from build123d import *

# Parameters (mm, degrees)
SKETCH_R         = 1.65
EXTRUDE_DEPTH    = 5
SKETCH001_W      = 50.041317
SKETCH001_H      = 10.034617
EXTRUDE001_DEPTH = 5


with BuildPart() as extrude_body:
    # Sketch → Extrude (new body)
    with BuildSketch(Plane.XY):
        Circle(SKETCH_R)
        with Locations((-10, 0)):
            Circle(SKETCH_R)
        with Locations((-20, 0)):
            Circle(SKETCH_R)
        with Locations((10, 0)):
            Circle(SKETCH_R)
        with Locations((20, 0)):
            Circle(SKETCH_R)
    extrude(amount=EXTRUDE_DEPTH)


with BuildPart() as cut:
    # Sketch001 → Extrude001 (new body)
    with BuildSketch(Plane.XY):
        with Locations((-0.018242, 0.017349)):
            Rectangle(SKETCH001_W, SKETCH001_H)
    extrude(amount=EXTRUDE001_DEPTH)

    # Cut: cut Extrude body
    add(extrude_body.part, mode=Mode.SUBTRACT)


solid = cut.part
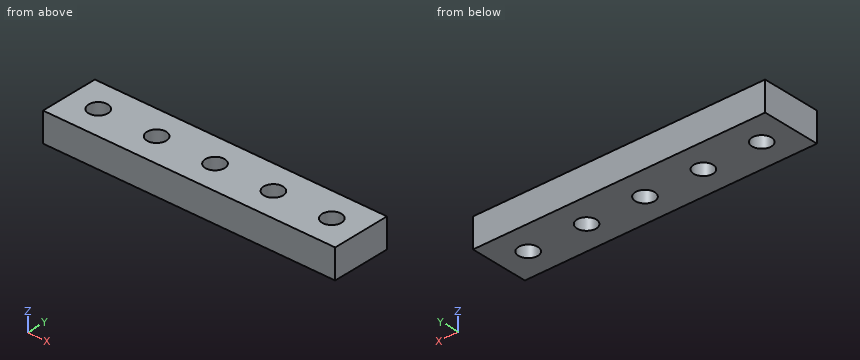
The model under review builds one solid part; all positions refer to its coordinate system, in mm. Give positions to 0.01 mm unless a question says otherwise; leave off trailing zeros. Loops run counter-clockwise (first coordinate to the right, second up) from the corner with the lowest first, then second, coordinate; pieces in that order, holes last. Notation, with made-up numbers: (-11.75, 44) -> (35.25, 44) arc R17 cw to (35.25, 74) -> close; hole circle Ø3 at (65, 27). An arc over 180 degrees is marked (long way). Put each result on its own line as item: value. Start each with the question number.
1. We need section B-B on z = 1.35. State the section outline as (x, y) points.
2. Wall thickness on probe 1 along Y at (x, z) = (10, 3); probe 2 along X at (y, z) = (-1.5, 4.65); probe 3 along Y at (x, z) = (1.5, 2.8): over which ranges is each line inside the solid? List them lowest first.
3. We need section C-C on x = 20. State the section outline as (y, z) points.
4. We need section A-A on y = 0. State the section outline as (x, z) points, then the cut area to 3 significant figures.
5. We need section D-D on x = -9.5. State the section outline as (y, z) points.
Determined:
1. outline: (-25.04, -5) -> (25, -5) -> (25, 5.03) -> (-25.04, 5.03) -> close; hole circle Ø3.3 at (-20, 0); hole circle Ø3.3 at (-10, 0); hole circle Ø3.3 at (0, 0); hole circle Ø3.3 at (10, 0); hole circle Ø3.3 at (20, 0)
2. probe 1: -5 to -1.65, 1.65 to 5.03
2. probe 2: -25.04 to -20.69, -19.31 to -10.69, -9.31 to -0.69, 0.69 to 9.31, 10.69 to 19.31, 20.69 to 25
2. probe 3: -5 to -0.69, 0.69 to 5.03
3. outline: (-5, 0) -> (-1.65, 0) -> (-1.65, 5) -> (-5, 5) -> close; (1.65, 0) -> (5.03, 0) -> (5.03, 5) -> (1.65, 5) -> close
4. outline: (-25.04, 0) -> (-21.65, 0) -> (-21.65, 5) -> (-25.04, 5) -> close; (-18.35, 0) -> (-11.65, 0) -> (-11.65, 5) -> (-18.35, 5) -> close; (-8.35, 0) -> (-1.65, 0) -> (-1.65, 5) -> (-8.35, 5) -> close; (1.65, 0) -> (8.35, 0) -> (8.35, 5) -> (1.65, 5) -> close; (11.65, 0) -> (18.35, 0) -> (18.35, 5) -> (11.65, 5) -> close; (21.65, 0) -> (25, 0) -> (25, 5) -> (21.65, 5) -> close
4. area: 168 mm^2
5. outline: (-5, 0) -> (-1.57, 0) -> (-1.57, 5) -> (-5, 5) -> close; (1.57, 0) -> (5.03, 0) -> (5.03, 5) -> (1.57, 5) -> close
